Autodesk Fusion 360 part; units mm, degrees
sketch "Sketch1" plane through (0, 0, 0) normal (0, 0, 1) x (1, 0, 0)
  line L0 (0, 0) -> (180, 0)
  line L1 (180, 0) -> (180, -12)
  line L2 (180, -12) -> (0, -12)
  line L3 (0, -12) -> (0, 0)
  dimension "d16" = 180
  dimension "d17" = 12
extrude "Extrude1" add sketch "Sketch1" along normal blind 10
sketch "Sketch6" plane through (0, 0, 10) normal (0, 0, 1) x (-1, 0, 0)
  line L0 (0, 12) -> (-180, 12)
  line L1 (-180, 12) -> (-180, 0)
  line L2 (-180, 0) -> (0, 0)
  line L3 (0, 0) -> (0, 12)
  circle A0 centre (-4.5, 6) radius 1.5
  circle A1 centre (-4.5, 6) radius 2.5
  circle A2 centre (-175.5, 6) radius 1.5
  circle A3 centre (-175.5, 6) radius 2.5
  line L4 (0, 12) -> (0, 0)
  line L5 (0, 0) -> (-180, 0)
  line L6 (-180, 0) -> (-180, 12)
  dimension "d65" = 3
  dimension "d66" = 1
  dimension "d67" = 3
  dimension "d68" = 1
  dimension "d69" = 4.5
  dimension "d70" = 6
  dimension "d71" = 4.5
  dimension "d72" = 6
extrude "Extrude9" cut sketch "Sketch6" against normal blind 100 contours A2
extrude "Extrude10" cut sketch "Sketch6" against normal blind 4 contours A3
extrude "Extrude11" cut sketch "Sketch6" against normal blind 100 contours A0
extrude "Extrude12" cut sketch "Sketch6" against normal blind 4 contours A1
equation "length = 180 mm"
equation "height = 10 mm"
equation "width = 12 mm"
equation "d16 = length"
equation "d17 = width"
equation "d18 = height"
equation "extra = 100 mm"
equation "bearing_outer_radius = 2.5 mm"
equation "bearing_width = 4 mm"
equation "bearing_big_distance = 2 mm + bearing_outer_radius"
equation "bearing_small_distance = width / 2"
equation "bearing_inner_radius = 1.5 mm"
equation "d65 = bearing_inner_radius * 2"
equation "d66 = bearing_outer_radius - bearing_inner_radius"
equation "d67 = bearing_inner_radius * 2"
equation "d68 = bearing_outer_radius - bearing_inner_radius"
equation "d69 = bearing_big_distance"
equation "d70 = bearing_small_distance"
equation "d71 = bearing_big_distance"
equation "d72 = bearing_small_distance"
Source: CAD feature listing. Evaluate the final solid. Frame: model axes, mm. A direction names the side the tool comes from. Coordinates: 2 decimals unless noted, no trailing zeros. Loops run counter-clockwise (first coordinate to the right, second up) from the corner with the lowest first, then second, coordinate; pieces in that order, holes last. Notation, with made-up numbers: (56, -23.75) -> (77, -23.75) arc R20 ccw to (77, 15.25) -> close; hole circle Ø8 at (71.5, -16). An arc over 180 degrees is marked (long way). Answer in a Markdown table with one row per item. Add a question column.
Q1. Section A-A on x = 4.5. Return the cut outline in (y, z), and give its area (3 significant figures).
Q2. Section B-B on y = -6. Return the cut outline in (x, z).
Q3. Reachability of faces 5 (the face through (2.115, -6.751, 8.028)), 6 (the face through (89, -6, 10)) from +Z, -Z, +X, -X, +Y, -Y: full face, straight path, thin tool, end or side. Return the list, or none.
Q4. Pull-direction query (X, two-part tool) for faces 1 (the face through (3, -5, 6)), 2 (the face through (180, -6, 5)), 3 (the face through (174, -5, 6)), 4 (the face through (89, 0, 5)); classes: pulls with the +X half, pulls with the -X half, needs draft (parallel to the pull), parting line crosses it, or undercut.
Q5. Ray query, line 1 along X through (y, z) = (-6, 7.9); line 2 along X through (y, z) = (-6, 2.45); line 3 along Y through (x, z) = (175.5, 8.85). Return the intervals inside material, ascending.
Q6. Section C-C on z = 7.5. Return the cut outline in (x, y), and give its area (3 significant figures).
Q7. Contact query for a flat-ended pin moving along its axis: pin 1 Ø2.5 at (x, y) = (4.5, -5.5) entering from +Z. Output: stop coordinate, or through.
Computed values:
| question | item | result |
|---|---|---|
| 1 | outline | (-12, 0) -> (-7.5, 0) -> (-7.5, 6) -> (-8.5, 6) -> (-8.5, 10) -> (-12, 10) -> close; (-4.5, 0) -> (0, 0) -> (0, 10) -> (-3.5, 10) -> (-3.5, 6) -> (-4.5, 6) -> close |
| 1 | area | 82.0 mm^2 |
| 2 | outline | (0, 0) -> (3, 0) -> (3, 6) -> (2, 6) -> (2, 10) -> (0, 10) -> close; (6, 0) -> (174, 0) -> (174, 6) -> (173, 6) -> (173, 10) -> (7, 10) -> (7, 6) -> (6, 6) -> close; (177, 0) -> (180, 0) -> (180, 10) -> (178, 10) -> (178, 6) -> (177, 6) -> close |
| 3 | face 5 | +Z |
| 3 | face 6 | +Z, +X, -X, +Y, -Y |
| 4 | face 1 | undercut |
| 4 | face 2 | pulls with the +X half |
| 4 | face 3 | undercut |
| 4 | face 4 | needs draft |
| 5 | line 1 | x = 0 to 2, 7 to 173, 178 to 180 |
| 5 | line 2 | x = 0 to 3, 6 to 174, 177 to 180 |
| 5 | line 3 | y = -12 to -8.5, -3.5 to 0 |
| 6 | outline | (0, -12) -> (180, -12) -> (180, 0) -> (0, 0) -> close; hole circle Ø5 at (4.5, -6); hole circle Ø5 at (175.5, -6) |
| 6 | area | 2,120 mm^2 |
| 7 | pin 1 | stops at z = 6 |
